Geometry check sheet. Reference: drawing and pictorial views, mm from the part's lowest x, y, z. A direction names the side the tool comes from. Round coordinates to 2 decimals unless told otherwise and drop trailing zeros. Write each loop counter-clockwise with the first axis right and the second up, starting at its lowest first coordinate (ties: lowest second). Pieces come first, ordered by that corner, then holes. Notation, with made-up numbers: M -30,-25 L -10,-25 A11 cw -10,-14 Z; hole C -5.75,58.25 d5. An arc over 180 degrees is marked long. One line per question, with ' | ' between items.
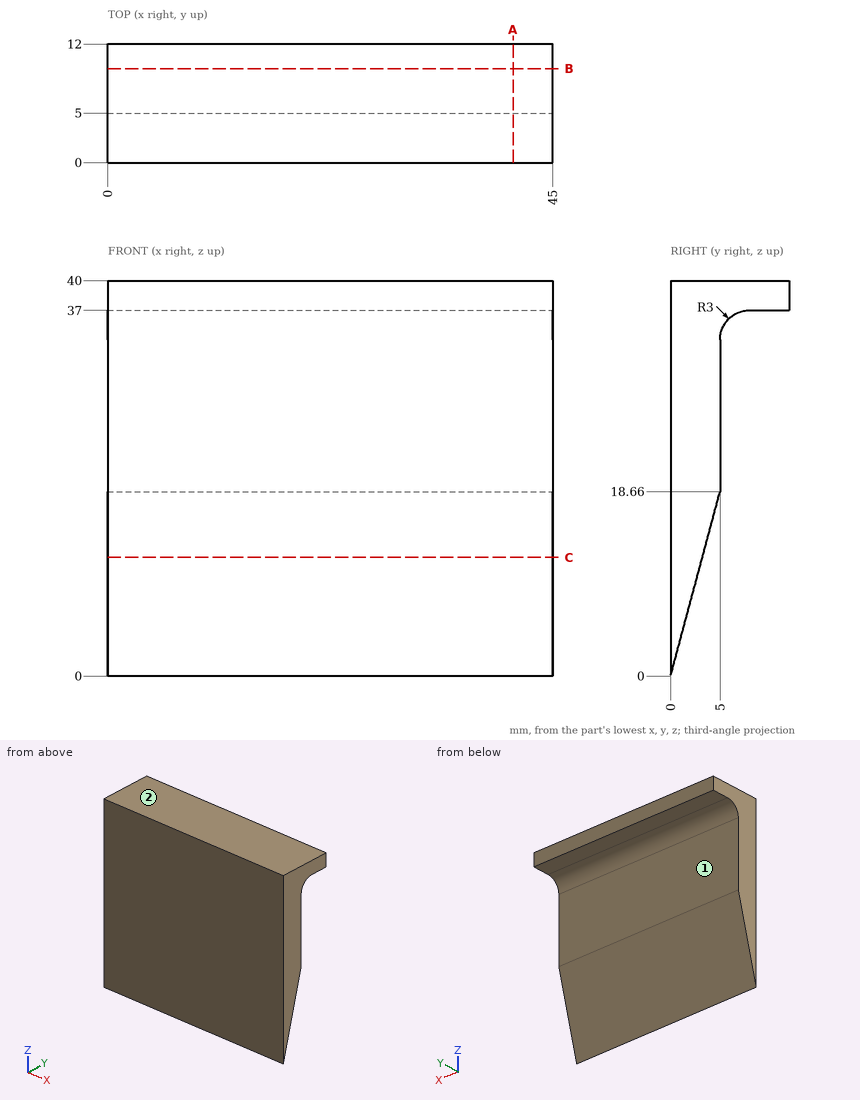
1. Section check C-C, the plane z = 12. Record the cut outline in (x, y) (1 decimal).
Results:
outline: M 0,0 L 45,0 L 45,3.2 L 0,3.2 Z
2. Section check B-B, the plane y = 9.5. Record the cut outline in (x, z), then the cut area to 3 significant figures.
Results:
outline: M 0,37 L 45,37 L 45,40 L 0,40 Z | area: 135 mm2
3. Thickness scan on line 1 (Z direction, x = 3.5, y = 9); line 2 (Y direction, x = 32, z = 31); line 3 (Y direction, x = 4.5, z = 6.5). Record the ranges inside material, lowest first.
Results:
line 1: z = 37 to 40 | line 2: y = 0 to 5 | line 3: y = 0 to 1.74
4. Section check A-A, the plane x = 41. Record the cut outline in (y, z), then the cut area to 3 significant figures.
Results:
outline: M 0,0 L 5,18.66 L 5,34 A3 cw 8,37 L 12,37 L 12,40 L 0,40 Z | area: 176 mm2
5. Tool access check on the marked faces 1 and 2. Record the directions out of +Z, -Z, +X, -X, +Y, -Y that give a thin tool (end or side, any length) a straight path to the whole face; none if there is none.
Results:
face 1: -Z, +X, -X, +Y | face 2: +Z, +X, -X, +Y, -Y
6. Go/stop test with flat-tipped pins: P1, Ø8, axis at x = 11.5, z = 15, coming from the +Y side; P2, Ø1.5, axis at y = 7, z = 22.5, coming from the +X side; P3, Ø1, axis at x = 7, z = 11, coming from the +Y side; P4, Ø4.5, axis at x = 23.5, y = 9.5, coming from the -Z side (1 decimal). Record where each tip stops, or that it passes through.
Results:
P1: stops at y = 5 | P2: passes through | P3: stops at y = 3.08 | P4: stops at z = 36.9
